The listing builds one solid part. Answer for the finished solid, in the listing's coordinates (mm). A direction names the side the tool comes from. Coordinates: 2 decimals unless noted, no trailing zeros. Loops run counter-clockwise (first coordinate to the right, second up) from the corner with the lowest first, then second, coordinate; pieces in that order, holes last. Notation, with made-up numbers: M 42,66 L 53,66 A15 ccw 53,72 Z; hole C 45,33 d8. An arc over 180 degrees is marked long. Answer in a Markdown table with one row per item. Add a question column.
Autodesk Inventor part; units mm, degrees
ref_plane "YZ Plane" through (0, 0, 0) normal (1, 0, 0) x (0, 1, 0)
ref_plane "XZ Plane" through (0, 0, 0) normal (0, 1, 0) x (-1, 0, 0)
ref_plane "XY Plane" through (0, 0, 0) normal (0, 0, 1) x (1, 0, 0)
sketch "Skizze1" plane through (0, 0, 0) normal (0, 0, 1) x (1, 0, 0)
  line L0 (-55, 75) -> (55, 75)
  line L1 (55, 75) -> (55, -75)
  line L2 (55, -75) -> (-55, -75) construction
  line L3 (-55, -75) -> (-55, 75)
  line L4 (0, -221.26) -> (0, 172.56) construction
  line L5 (-81, 0) -> (101, 0) construction
  line L6 (55, -75) -> (-16, -75) construction
  line L7 (-16, -75) -> (-16, -165) construction
  line L8 (-16, -165) -> (55, -165)
  line L9 (55, -165) -> (55, -75)
  line L10 (55, -165) -> (75, -165)
  line L11 (75, -165) -> (75, 116.3)
  line L12 (75, 116.3) -> (55, 116.3)
  line L13 (55, 116.3) -> (55, -165) construction
  line L14 (-55, -75) -> (-16, -75) construction
  line L15 (-16, -75) -> (-16, -99) construction
  line L16 (-16, -99) -> (-55, -99)
  line L17 (-55, -99) -> (-55, -75)
  line L18 (-16, -99) -> (-16, -165)
  line L19 (55, 116.3) -> (35, 116.3)
  line L20 (35, 116.3) -> (35, 75)
  line L21 (35, 75) -> (55, 75)
  line L22 (55, 75) -> (55, 116.3) construction
  point P0 (0, 0)
  point P1 (-35.5, -75)
  dimension "d0" = 110
  dimension "d1" = 150
  dimension "d4" = 90
  dimension "d5" = 71
  dimension "d6" = 281.3
  dimension "d7" = 20
  dimension "d139" = 24
  dimension "d140" = 20
extrude "Extrusion1" add sketch "Skizze1" along normal blind 2.5
sketch "Skizze7" plane through (0, 0, 2.5) normal (0, 0, 1) x (1, 0, 0)
  line L0 (75, 116.3) -> (35, 116.3)
  line L1 (75, 116.3) -> (73.5, 116.3)
  line L2 (73.5, 116.3) -> (73.5, -165) construction
  line L3 (73.5, -165) -> (75, -165)
  line L4 (75, -165) -> (75, 116.3)
  line L5 (75, 90.67) -> (73.5, 90.67)
  line L6 (73.5, 90.67) -> (73.5, 85.67)
  line L7 (73.5, 85.67) -> (75, 85.67)
  line L8 (75, 85.67) -> (75, 90.67)
  line L9 (75, -134.37) -> (73.5, -134.37)
  line L10 (73.5, -134.37) -> (73.5, -139.37)
  line L11 (73.5, -139.37) -> (75, -139.37)
  line L12 (75, -139.37) -> (75, -134.37)
  line L13 (-16, -165) -> (75, -165)
  line L14 (75, -165) -> (75, 116.3)
  line L15 (75, -26.85) -> (73.5, -26.85)
  line L16 (73.5, -26.85) -> (73.5, -21.85)
  line L17 (73.5, -21.85) -> (75, -21.85)
  line L18 (75, -21.85) -> (75, -26.85)
  point P0 (0, 0)
  point P1 (45.75, 136.3)
  point P2 (-15.25, -145)
  point P3 (75, 85.67)
  point P4 (49.25, 116.3)
  point P5 (74.25, -165)
  point P6 (75, -26.85)
  point P7 (75, -21.85)
  dimension "d66" = 1.5
  dimension "d67" = 5
  dimension "d68" = 25.63
  dimension "d69" = 25.63
  dimension "d70" = 5
  dimension "d156" = 5
  dimension "d157" = 138.15
extrude "Extrusion6" add sketch "Skizze7" along normal blind 5
sketch "Skizze8" plane through (73.5, -139.37, 2.5) normal (-1, 0, 0) x (0, 0, 1)
  line L0 (0, 0) -> (5, 0)
  line L1 (5, 5) -> (5, 0)
  line L2 (0, 225.04) -> (5, 225.04)
  line L3 (5, 230.04) -> (5, 225.04)
  line L4 (0, 230.04) -> (5, 230.04)
  line L5 (0, 225.04) -> (0, 230.04)
  line L6 (5, 112.52) -> (5, 117.52)
  line L7 (0, 112.52) -> (5, 112.52)
  point P0 (-2.5, 139.37)
  point P1 (1.5, 2.5)
  point P2 (2.5, 0)
  point P3 (1.5, 227.54)
  point P4 (2.5, 115.02)
  dimension "d73" = 2.5
  dimension "d74" = 3.5
  dimension "d75" = 3.5
  dimension "d76" = 2.5
  dimension "d158" = 2.5
  dimension "d159" = 2.5
hole "Bohrung1" at (73.5, 88.17, 4) at (73.5, -136.87, 4) at (73.5, -24.35, 5) direction (1, 0, 0) diameter 3 depth 1.5
sketch "Skizze15" plane through (0, 0, 2.5) normal (0, 0, 1) x (1, 0, 0)
  line L0 (73.5, -134.37) -> (75, -134.37)
  line L1 (75, -134.37) -> (75, -26.85)
  line L2 (75, 85.67) -> (73.5, 85.67)
  line L3 (73.5, 85.67) -> (73.5, 88.17)
  line L4 (73.5, 88.17) -> (73.5, 90.67)
  line L5 (73.5, 90.67) -> (75, 90.67)
  line L6 (75, 90.67) -> (75, 116.3)
  line L7 (75, 116.3) -> (35, 116.3)
  line L8 (35, 116.3) -> (35, 75)
  line L9 (35, 75) -> (-55, 75)
  line L10 (-55, 75) -> (-55, -99)
  line L11 (-55, -99) -> (-16, -99)
  line L12 (-16, -99) -> (-16, -165)
  line L13 (-16, -165) -> (75, -165)
  line L14 (75, -165) -> (75, -139.37)
  line L15 (75, -139.37) -> (73.5, -139.37)
  line L16 (73.5, -139.37) -> (73.5, -136.87)
  line L17 (73.5, -136.87) -> (73.5, -134.37)
  line L18 (75, 116.3) -> (35, 116.3)
  line L19 (36.5, 116.3) -> (36.5, 73.5)
  line L20 (36.5, 73.5) -> (-23, 73.5)
  line L21 (-23, 73.5) -> (-23, 75)
  line L22 (-37, 75) -> (-37, 73.5)
  line L23 (-37, 73.5) -> (-53.5, 73.5)
  line L24 (-53.5, 73.5) -> (-53.5, -97.5)
  line L25 (-53.5, -97.5) -> (-14.5, -97.5)
  line L26 (-14.5, -97.5) -> (-14.5, -99)
  line L27 (-14.5, -99) -> (-16, -99)
  line L28 (-14.5, -131) -> (-14.5, -163.5)
  line L29 (-14.5, -163.5) -> (-12, -163.5)
  line L30 (-12, -163.5) -> (-12, -165)
  line L31 (48, -165) -> (48, -163.5)
  line L32 (48, -163.5) -> (75, -163.5)
  line L33 (-14.5, -131) -> (-16, -131)
  line L34 (75, -26.85) -> (73.5, -26.85)
  line L35 (73.5, -26.85) -> (73.5, -21.85)
  line L36 (73.5, -21.85) -> (75, -21.85)
  line L37 (75, -21.85) -> (75, 85.67)
  line L38 (75, 111.3) -> (75, 116.3)
  line L39 (75, -163.5) -> (73.5, -163.5)
  line L40 (73.5, -163.5) -> (73.5, -158.5)
  line L41 (73.5, -158.5) -> (75, -158.5)
  line L42 (75, -158.5) -> (75, -163.5)
  line L43 (73.5, 114.8) -> (68.5, 114.8)
  line L44 (68.5, 114.8) -> (68.5, 109.8)
  line L45 (68.5, 109.8) -> (73.5, 109.8)
  line L46 (73.5, 109.8) -> (73.5, 114.8)
  point P0 (0, 0)
  point P1 (75, -158.5)
  dimension "d141" = 1.5
  dimension "d142" = 1.5
  dimension "d143" = 1.5
  dimension "d144" = 1.5
  dimension "d145" = 1.5
  dimension "d146" = 1.5
  dimension "d147" = 4
  dimension "d148" = 64
  dimension "d149" = 0
  dimension "d150" = 32
  dimension "d151" = 18
  dimension "d152" = 14
  dimension "d171" = 5
  dimension "d172" = 1.5
  dimension "d224" = 5
  dimension "d225" = 5
  dimension "d226" = 1.5
  dimension "d227" = 1.5
extrude "Extrusion13" add sketch "Skizze15" along normal blind 26 contours L14 L32 L40 L41 | L14 L13 L31 L32 | L13 L12 L33 L28 L29 L30 | L11 L10 L9 L22 L23 L24 L25 L26 L27 | L19 L20 L21 L9 L8 L7 | L46 L45 L44 L43
fillet "Rundung1" radius 2 4 edges at (35, 75, 14.25) (-55, 75, 14.25) (-55, -99, 14.25) (-16, -165, 14.25)
sketch "Skizze16" plane through (-55, -97, 0) normal (-1, 0, 0) x (0, 0, 1)
  line L0 (18.35, 76.1) -> (10.15, 76.1)
  line L1 (10.15, 76.1) -> (10.15, 60)
  line L2 (10.15, 60) -> (18.35, 60)
  line L3 (18.35, 60) -> (18.35, 76.1)
  circle A0 centre (14.25, 35) radius 3.5
  line L4 (0, 170) -> (28.5, 170)
  line L5 (0, 170) -> (0, 0)
  line L6 (28.5, 0) -> (0, 0)
  line L7 (28.5, 170) -> (28.5, 0)
  point P0 (0, 97)
  dimension "d160" = 16.1
  dimension "d161" = 8.2
  dimension "d162" = 7
  dimension "d163" = 14.25
  dimension "d164" = 35
  dimension "d165" = 60
  dimension "d166" = 10.15
extrude "Extrusion14" cut sketch "Skizze16" against normal up to surface (1.5 mm away) contours L3 L2 L1 L0 | A0
sketch "Skizze17" plane through (0, 0, 28.5) normal (0, 0, 1) x (1, 0, 0)
  line L0 (73.5, -163.5) -> (48, -163.5)
  line L1 (73.5, -163.5) -> (68.5, -163.5)
  line L2 (68.5, -163.5) -> (68.5, -158.5)
  line L3 (68.5, -158.5) -> (73.5, -158.5)
  line L4 (73.5, -158.5) -> (73.5, -163.5)
  line L5 (-14.5, -131) -> (-14.5, -163.5)
  line L6 (-14.5, -163.5) -> (-9.5, -163.5)
  line L7 (-9.5, -163.5) -> (-9.5, -158.5)
  line L8 (-9.5, -158.5) -> (-14.5, -158.5)
  line L9 (-14.5, -158.5) -> (-14.5, -163.5)
  line L10 (-53.5, 73.5) -> (-53.5, -97.5)
  line L11 (-53.5, -97.5) -> (-48.5, -97.5)
  line L12 (-48.5, -97.5) -> (-48.5, -92.5)
  line L13 (-48.5, -92.5) -> (-53.5, -92.5)
  line L14 (-53.5, -92.5) -> (-53.5, -97.5)
  line L15 (-53.5, 73.5) -> (-48.5, 73.5)
  line L16 (-48.5, 73.5) -> (-48.5, 68.5)
  line L17 (-48.5, 68.5) -> (-53.5, 68.5)
  line L18 (-53.5, 68.5) -> (-53.5, 73.5)
  line L19 (36.5, 73.5) -> (36.5, 116.3)
  line L20 (36.5, 73.5) -> (31.5, 73.5)
  line L21 (31.5, 73.5) -> (31.5, 68.5)
  line L22 (31.5, 68.5) -> (36.5, 68.5)
  line L23 (36.5, 68.5) -> (36.5, 73.5)
  point P0 (0, 0)
  point P1 (-14.5, -158.5)
  dimension "d173" = 5
  dimension "d174" = 5
  dimension "d175" = 5
  dimension "d176" = 5
  dimension "d177" = 5
  dimension "d178" = 5
  dimension "d179" = 5
  dimension "d180" = 5
  dimension "d181" = 5
  dimension "d182" = 5
extrude "Extrusion15" add sketch "Skizze17" against normal blind 5
sketch "Skizze19" plane through (0, 0, 28.5) normal (0, 0, 1) x (1, 0, 0)
  line L0 (-14, -165) -> (75, -165)
  line L1 (75, -165) -> (75, -158.5)
  line L2 (-12, -165) -> (48, -165)
  line L3 (-16, -131) -> (-16, -163)
  line L4 (-53, -99) -> (-14.5, -99)
  line L5 (-55, 73) -> (-55, -97)
  line L6 (33, 75) -> (-53, 75)
  line L7 (33, 75) -> (-53, 75)
  line L8 (31.5, 73.5) -> (31.5, 68.5)
  line L9 (36.5, 116.3) -> (35, 116.3)
  line L10 (75, 90.67) -> (75, 116.3)
  point P0 (0, 0)
  point P1 (71, -161)
  point P2 (-12, -161)
  point P3 (-51, -95)
  point P4 (-51, 71)
  point P5 (34, 71)
  point P6 (71, 112.3)
  point P7 (-16, -163)
  point P8 (-37, 75)
  point P9 (-23, 75)
  point P10 (69.25, -139.37)
  point P11 (-21.75, -99)
  dimension "d205" = 4
  dimension "d206" = 4
  dimension "d207" = 4
  dimension "d208" = 4
  dimension "d209" = 4
  dimension "d210" = 4
  dimension "d211" = 4
  dimension "d212" = 4
  dimension "d213" = 4
  dimension "d214" = 2.5
  dimension "d215" = 4
  dimension "d228" = 4
hole "Bohrung3" at (71, -161, 28.5) at (-12, -161, 28.5) at (-51, -95, 28.5) at (71, 112.3, 28.5) at (34, 71, 28.5) at (-51, 71, 28.5) direction (0, 0, -1) diameter 2 depth 5
properties part number "PCB_Grundplatte_Platinengehäuse_V2"
(1) The mould has two halves that part along X. Classify faces 6 (the face through (31.5, 71, 26)), 7 (the face through (75, -56, 2)), 8 (the face through (-51, -92.5, 26)): released by +X, released by -X, zero draft, split by the parting line, or undercut.
(2) A cutting plane is placed at A-A (y = 11). Give the vertices of the cut face in (x, z).
(3) For faces 1 (the face through (73.5, -137, 6)), 2 (the face through (-9.5, -161, 26)), 3 (the face through (68.5, 112, 15)), 4 (the face through (-12, -158.5, 26)), 5 (the face through (-45, 73.5, 15)), determine the directions among +Z, -Z, +X, -X, +Y, -Y from which every point of the face is accessible in a straight line to the end or side of a thin tool.
(4) Each of these flat-tipped pins is pushed along its axis until it touches: pin 1 (13 mm diameter, centred on x = -45.5, z = 18, fed in from -Y); pin 2 (8 mm diameter, centred on y = -141.5, z = 22, fed in from +X); pin 3 (5 mm diameter, centred on x = 70.5, z = 22, fed in from +Y). Where does it stop, or does it pass through?
(5) A cutting plane is placed at B-B (x = -1.5). Give the vertices of the cut face in (y, z), plus the area to 3 significant figures.
(6) Straight lines are drawn through the part: line 1 (X direction, y = -161, z = 25.9); line 2 (Y direction, x = -51, z = 26.8); line 3 (Y direction, x = 71, z = 25.2). For each, find the intervals that lie inside material, in ascending order.
Solved:
| question | item | result |
|---|---|---|
| 1 | face 6 | undercut |
| 1 | face 7 | released by +X |
| 1 | face 8 | zero draft |
| 2 | outline | M -55,0 L 75,0 L 75,2.5 L -53.5,2.5 L -53.5,28.5 L -55,28.5 Z |
| 3 | face 1 | +Z |
| 3 | face 2 | +Z, -Y |
| 3 | face 3 | +Z, +Y |
| 3 | face 4 | +Z, +X |
| 3 | face 5 | none |
| 4 | pin 1 | stops at y = -99 |
| 4 | pin 2 | stops at x = -14.5 |
| 4 | pin 3 | stops at y = 114.8 |
| 5 | outline | M -165,0 L 75,0 L 75,28.5 L 73.5,28.5 L 73.5,2.5 L -165,2.5 Z |
| 5 | area | 639 mm² |
| 6 | line 1 | x = -16 to -13, -11 to -9.5, 68.5 to 70, 72 to 75 |
| 6 | line 2 | y = -99 to -96, -94 to -92.5, 68.5 to 70, 72 to 75 |
| 6 | line 3 | y = -165 to -162, -160 to -158.5, 109.8 to 111.3, 113.3 to 114.8 |
